Could you check a few things on this model? Use its own coordinates, in mm. A direction names the side the tool comes from. Coordinates: 2 decimals unless noted, no trailing zeros. Loops run counter-clockwise (first coordinate to the right, second up) from the corner with the lowest first, then second, coordinate; pieces in that order, holes last. Notation, with made-up numbers: (-15.75, 47.25) -> (32.25, 47.25) arc R13 cw to (32.25, 70.25) -> close; hole circle Ø4 at (9.25, 18). An arc over 180 degrees is marked (long way). One line per question, with ' | ' between items. Start each with the question number.
(1) Suppose I cut it at C-C (z = 31.5). Please give me the cut outline in (x, y) (3 decimals).
(2) Suppose I cut it at D-D (x = 34.29). Please give me the cut outline in (y, z) (3 decimals), plus the area to 3 significant figures.
(3) Suppose I cut it at B-B (y = 21.59). Please give me the cut outline in (x, z) (3 decimals).
(4) If I drill on line 1 along X through (y, z) = (37, 16.5); line 2 along Y through (x, z) = (53.29, 28); line 3 along Y through (x, z) = (46, 22), over which ranges is the centre line in solid material (lowest first)?
(5) Suppose I cut it at A-A (x = 53.29). Please give me the cut outline in (y, z) (3 decimals).
(6) Which directions (+Z, -Z, +X, -X, +Y, -Y) give clear straight access to the entire face, cutting with the end or side of a thin tool? Please do faces 1 (the face through (68.58, 21, 13)), 2 (the face through (66.407, 2.291, 12.522)), 3 (the face through (2.173, 40.889, 12.522)), 4 (the face through (35, 43.18, 13)), 5 (the face through (66.289, 41.007, 12.522)).
(7) I'm going to push flat-ended pins straight in: pin 1 Ø4 at (x, z) = (12.5, 6) entering from -Y; pin 2 Ø7.5 at (y, z) = (27.5, 14) entering from +X; pin 3 Ø7.5 at (y, z) = (18.5, 9) entering from -X. Where does each tip first touch, or does it pass through?
(8) If we mould it in two halves opening along Y, with no side actions, what happens to faces 6 (the face through (46.03, 36.58, 19.32)), 7 (the face through (34, -3.81, 30)), 8 (the face through (72.39, 21, 30)), 9 (the face through (19.03, 6.755, 19.317))? For each: pulls with the +Y half, pulls with the -Y half, needs draft (parallel to the pull), parting line crosses it, or undercut.
Autodesk Inventor part; units mm, degrees
ref_plane "YZ Plane" through (0, 0, 0) normal (1, 0, 0) x (0, 1, 0)
ref_plane "XZ Plane" through (0, 0, 0) normal (0, 1, 0) x (-1, 0, 0)
ref_plane "XY Plane" through (0, 0, 0) normal (0, 0, 1) x (1, 0, 0)
sketch "Sketch1" plane through (0, 0, 0) normal (0, 0, 1) x (1, 0, 0)
  line L0 (7.62, 0) -> (60.96, 0)
  line L1 (68.58, 7.62) -> (68.58, 35.56)
  line L2 (60.96, 43.18) -> (7.62, 43.18)
  line L3 (0, 35.56) -> (0, 7.62)
  arc A0 (7.62, 43.18) -> (0, 35.56) centre (7.62, 35.56) ccw
  arc A1 (0, 7.62) -> (7.62, 0) centre (7.62, 7.62) ccw
  arc A2 (68.58, 35.56) -> (60.96, 43.18) centre (60.96, 35.56) ccw
  arc A3 (60.96, 0) -> (68.58, 7.62) centre (60.96, 7.62) ccw
  point P0 (0, 0)
  point P1 (68.58, 43.18)
  point P2 (68.58, 0)
  point P3 (0, 43.18)
  dimension "d0" = 68.58
  dimension "d1" = 43.18
  dimension "d3" = 7.62
extrude "Extrusion1" add sketch "Sketch1" along normal blind 25.4
sketch "Sketch2" plane through (0, 0, 25.4) normal (0, 0, 1) x (1, 0, 0)
  line L0 (2.54, -3.81) -> (66.04, -3.81)
  line L1 (72.39, 2.54) -> (72.39, 40.64)
  line L2 (66.04, 46.99) -> (2.54, 46.99)
  line L3 (-3.81, 40.64) -> (-3.81, 2.54)
  line L4 (60.96, 43.18) -> (7.62, 43.18) construction
  line L5 (0, 35.56) -> (0, 7.62) construction
  line L6 (7.62, 0) -> (60.96, 0) construction
  line L7 (68.58, 7.62) -> (68.58, 35.56) construction
  arc A0 (2.54, 46.99) -> (-3.81, 40.64) centre (2.54, 40.64) ccw
  arc A1 (-3.81, 2.54) -> (2.54, -3.81) centre (2.54, 2.54) ccw
  arc A2 (66.04, -3.81) -> (72.39, 2.54) centre (66.04, 2.54) ccw
  arc A3 (72.39, 40.64) -> (66.04, 46.99) centre (66.04, 40.64) ccw
  point P0 (0, 0)
  point P1 (72.39, 46.99)
  point P2 (72.39, -3.81)
  point P3 (-3.81, 46.99)
  point P4 (34.29, 46.99)
  point P5 (34.29, 43.18)
  point P6 (68.58, 21.59)
  point P7 (72.39, 21.59)
  dimension "d6" = 76.2
  dimension "d7" = 50.8
  dimension "d8" = 6.35
extrude "Extrusion2" add sketch "Sketch2" along normal blind 12.7
fillet "Fillet1" radius 3.175 8 edges at (-1.9501, 45.1301, 38.1) (-3.81, 21.59, 38.1) (-1.9501, -1.9501, 38.1) (34.29, -3.81, 38.1) (70.5301, -1.9501, 38.1) (72.39, 21.59, 38.1) (70.5301, 45.1301, 38.1) (34.29, 46.99, 38.1)
sketch "Sketch3" plane through (0, 0, 38.1) normal (0, 0, 1) x (1, 0, 0)
  circle A0 centre (34.29, 21.59) radius 14.5
  line L0 (-0.635, 2.54) -> (-0.635, 40.64) construction
  line L1 (2.54, 43.815) -> (66.04, 43.815) construction
  circle A1 centre (34.29, 21.59) radius 19 construction
  circle A2 centre (47.725, 35.025) radius 2.3
  circle A3 centre (15.29, 21.59) radius 2.3
  circle A4 centre (47.725, 8.155) radius 2.3
  circle A5 centre (53.29, 21.59) radius 2.3
  circle A6 centre (20.855, 35.025) radius 2.3
  circle A7 centre (20.855, 8.155) radius 2.3
  line L2 (20.855, 35.025) -> (34.29, 21.59) construction
  line L3 (34.29, 21.59) -> (15.29, 21.59) construction
  point P0 (0, 0)
  point P1 (34.29, 43.815)
  point P2 (-0.635, 21.59)
  dimension "d12" = 29
  dimension "d13" = 38
  dimension "d14" = 4.6
  dimension "d15" = 45
extrude "Extrusion3" cut sketch "Sketch3" against normal up to surface (38.1 mm away)
properties part number "2x3_Spacer"
Checks:
1) outline: (-3.81, 2.54) arc R6.35 ccw to (2.54, -3.81) -> (66.04, -3.81) arc R6.35 ccw to (72.39, 2.54) -> (72.39, 40.64) arc R6.35 ccw to (66.04, 46.99) -> (2.54, 46.99) arc R6.35 ccw to (-3.81, 40.64) -> close; hole circle Ø4.6 at (15.29, 21.59); hole circle Ø4.6 at (20.855, 8.155); hole circle Ø4.6 at (20.855, 35.025); hole circle Ø29 at (34.29, 21.59); hole circle Ø4.6 at (47.725, 8.155); hole circle Ø4.6 at (47.725, 35.025); hole circle Ø4.6 at (53.29, 21.59)
2) outline: (-3.81, 25.4) -> (0, 25.4) -> (0, 0) -> (7.09, 0) -> (7.09, 38.1) -> (-0.635, 38.1) arc R3.175 ccw to (-3.81, 34.925) -> close; (36.09, 0) -> (43.18, 0) -> (43.18, 25.4) -> (46.99, 25.4) -> (46.99, 34.925) arc R3.175 ccw to (43.815, 38.1) -> (36.09, 38.1) -> close | area: 633 mm^2
3) outline: (-3.81, 25.4) -> (0, 25.4) -> (0, 0) -> (12.99, 0) -> (12.99, 38.1) -> (-0.635, 38.1) arc R3.175 ccw to (-3.81, 34.925) -> close; (17.59, 0) -> (19.79, 0) -> (19.79, 38.1) -> (17.59, 38.1) -> close; (48.79, 0) -> (50.99, 0) -> (50.99, 38.1) -> (48.79, 38.1) -> close; (55.59, 0) -> (68.58, 0) -> (68.58, 25.4) -> (72.39, 25.4) -> (72.39, 34.925) arc R3.175 ccw to (69.215, 38.1) -> (55.59, 38.1) -> close
4) line 1: x = 0.14 to 19.68, 22.03 to 46.55, 48.9 to 68.44 | line 2: y = -3.81 to 19.29, 23.89 to 46.99 | line 3: y = 0 to 6.63, 9.68 to 13.04, 30.14 to 33.5, 36.55 to 43.18
5) outline: (-3.81, 25.4) -> (0, 25.4) -> (0, 0) -> (19.29, 0) -> (19.29, 38.1) -> (-0.635, 38.1) arc R3.175 ccw to (-3.81, 34.925) -> close; (23.89, 0) -> (43.18, 0) -> (43.18, 25.4) -> (46.99, 25.4) -> (46.99, 34.925) arc R3.175 ccw to (43.815, 38.1) -> (23.89, 38.1) -> close
6) face 1: -Z, +X, +Y, -Y | face 2: -Z, +X, -Y | face 3: -Z, -X, +Y | face 4: -Z, +X, -X, +Y | face 5: -Z, +X, +Y
7) pin 1: stops at y = 0 | pin 2: stops at x = 68.58 | pin 3: stops at x = 0
8) face 6: undercut | face 7: pulls with the -Y half | face 8: needs draft | face 9: undercut
